```python
from build123d import *

# Parameters (mm, degrees)
SKETCH1_W           = 35
SKETCH1_H           = 10
BOSS_EXTRUDE1_DEPTH = 70
SKETCH2_3_R         = 7.5
SKETCH2_3_R_2       = 5
BOSS_EXTRUDE2_DEPTH = 10
CUT_EXTRUDE1_START  = -70
SKETCH2_4_R         = 5
CUT_EXTRUDE1_DEPTH  = 70
SKETCH3_R           = 7.5
SKETCH3_R_2         = 5
BOSS_EXTRUDE3_DEPTH = 10
CUT_EXTRUDE3_START  = -10
SKETCH3_2_R         = 5
CUT_EXTRUDE3_DEPTH  = 10
BOSS_EXTRUDE6_START = 6
BOSS_EXTRUDE6_DEPTH = 6


with BuildPart() as part:
    # Sketch1 → Revolve1 (revolve)
    with BuildSketch(Plane(origin=(0, 0, 0), x_dir=(0, 0, -1), z_dir=(1, 0, 0)), mode=Mode.PRIVATE) as revolve1_sk:
        Polygon((35, 79.538461538), (35, 89.538461538), (45, 89.538461538), (45, -20.461538462), (0, -20.461538462), (0, -10.461538462), (0, 49.538461538), (8, 49.538461538), (27, -10.461538462), (35, -10.461538462), align=None)
        with Locations((17.5, 84.538461538)):
            Rectangle(SKETCH1_W, SKETCH1_H)
    revolve(revolve1_sk.sketch.rotate(Axis((0, 0, 0), (0, -1, 0)), 180), axis=Axis((0, 0, 0), (0, -1, 0)))

    # Sketch2 → Boss-Extrude1 (add)
    with BuildSketch(Plane.XZ.offset(20.461538462)):
        with BuildLine():
            Line((40, 5), (10.356157589, 5))
            ThreePointArc((10.356157589, 5), (10.819851722, 3.896255731), (11.166285361, 2.750285665))
            Line((11.166285361, 2.750285665), (22.5, 1))
            Line((22.5, 1), (22.5, -1))
            Line((22.5, -1), (11.166285361, -2.750285665))
            ThreePointArc((11.166285361, -2.750285665), (10.819851722, -3.896255731), (10.356157589, -5))
            Line((10.356157589, -5), (40, -5))
            Line((40, -5), (40, 5))
        make_face()
        with BuildLine():
            ThreePointArc((2.750285665, 11.166285361), (3.896255731, 10.819851722), (5, 10.356157589))
            Line((5, 10.356157589), (5, 40))
            Line((5, 40), (-5, 40))
            Line((-5, 40), (-5, 10.356157589))
            ThreePointArc((-5, 10.356157589), (-3.896255731, 10.819851722), (-2.750285665, 11.166285361))
            Line((-2.750285665, 11.166285361), (-1, 22.5))
            Line((-1, 22.5), (1, 22.5))
            Line((1, 22.5), (2.750285665, 11.166285361))
        make_face()
        with BuildLine():
            Line((5, -40), (5, -10.356157589))
            ThreePointArc((5, -10.356157589), (3.896255731, -10.819851722), (2.750285665, -11.166285361))
            Line((2.750285665, -11.166285361), (1, -22.5))
            Line((1, -22.5), (-1, -22.5))
            Line((-1, -22.5), (-2.750285665, -11.166285361))
            ThreePointArc((-2.750285665, -11.166285361), (-3.896255731, -10.819851722), (-5, -10.356157589))
            Line((-5, -10.356157589), (-5, -40))
            Line((-5, -40), (5, -40))
        make_face()
        with BuildLine():
            ThreePointArc((-11.166285361, 2.750285665), (-10.819851722, 3.896255731), (-10.356157589, 5))
            Line((-10.356157589, 5), (-40, 5))
            Line((-40, 5), (-40, -5))
            Line((-40, -5), (-10.356157589, -5))
            ThreePointArc((-10.356157589, -5), (-10.819851722, -3.896255731), (-11.166285361, -2.750285665))
            Line((-11.166285361, -2.750285665), (-22.5, -1))
            Line((-22.5, -1), (-22.5, 1))
            Line((-22.5, 1), (-11.166285361, 2.750285665))
        make_face()
    extrude(amount=-BOSS_EXTRUDE1_DEPTH)

    # Sketch2<3> → Boss-Extrude2 (add)
    with BuildSketch(Plane.XZ.offset(20.461538462)):
        with Locations(Location((0, 0, 0), (0, 0, 270))):
            Circle(SKETCH2_3_R)
        with Locations(Location((0, 0, 0), (0, 0, 270))):
            Circle(SKETCH2_3_R_2, mode=Mode.SUBTRACT)
    extrude(amount=BOSS_EXTRUDE2_DEPTH)

    # Sketch2<4> → Cut-Extrude1 (cut)
    with BuildSketch(Plane.XZ.offset(20.461538462).offset(CUT_EXTRUDE1_START)):
        with Locations(Location((0, 0, 0), (0, 0, 270))):
            Circle(SKETCH2_4_R)
    extrude(amount=CUT_EXTRUDE1_DEPTH, mode=Mode.SUBTRACT)

    # Sketch3 → Boss-Extrude3 (add)
    with BuildSketch(Plane(origin=(0, 89.538461538, 0), x_dir=(1, 0, 0), z_dir=(0, 1, 0))):
        with Locations(Location((22, 0, 0), (0, 0, 270))):
            Circle(SKETCH3_R)
        with Locations(Location((22, 0, 0), (0, 0, 270))):
            Circle(SKETCH3_R_2, mode=Mode.SUBTRACT)
    extrude(amount=BOSS_EXTRUDE3_DEPTH)

    # Sketch3<2> → Cut-Extrude3 (cut)
    with BuildSketch(Plane(origin=(0, 89.538461538, 0), x_dir=(1, 0, 0), z_dir=(0, 1, 0)).offset(CUT_EXTRUDE3_START)):
        with Locations(Location((22, 0, 0), (0, 0, 270))):
            Circle(SKETCH3_2_R)
    extrude(amount=CUT_EXTRUDE3_DEPTH, mode=Mode.SUBTRACT)

    # Sketch2<5> → Boss-Extrude6 (add)
    with BuildSketch(Plane.XZ.offset(20.461538462).offset(BOSS_EXTRUDE6_START)):
        with BuildLine():
            ThreePointArc((-9.840501743, 5.951010455), (-8.131727984, 8.131727984), (-5.951010455, 9.840501743))
            Line((-5.951010455, 9.840501743), (-15.202795796, 16.617009358))
            Line((-15.202795796, 16.617009358), (-15.909902577, 15.909902577))
            Line((-15.909902577, 15.909902577), (-16.617009358, 15.202795796))
            Line((-16.617009358, 15.202795796), (-9.840501743, 5.951010455))
        make_face()
        with BuildLine():
            ThreePointArc((-2.750285665, 11.166285361), (0, 11.5), (2.750285665, 11.166285361))
            Line((2.750285665, 11.166285361), (1, 22.5))
            Line((1, 22.5), (0, 22.5))
            Line((0, 22.5), (-1, 22.5))
            Line((-1, 22.5), (-2.750285665, 11.166285361))
        make_face()
        with BuildLine():
            ThreePointArc((5.951010455, 9.840501743), (8.131727984, 8.131727984), (9.840501743, 5.951010455))
            Line((9.840501743, 5.951010455), (16.617009358, 15.202795796))
            Line((16.617009358, 15.202795796), (15.909902577, 15.909902577))
            Line((15.909902577, 15.909902577), (15.202795796, 16.617009358))
            Line((15.202795796, 16.617009358), (5.951010455, 9.840501743))
        make_face()
        with BuildLine():
            Line((22.5, 1), (11.166285361, 2.750285665))
            ThreePointArc((11.166285361, 2.750285665), (11.416266501, 1.385228925), (11.5, 0))
            ThreePointArc((11.5, 0), (11.416266501, -1.385228925), (11.166285361, -2.750285665))
            Line((11.166285361, -2.750285665), (22.5, -1))
            Line((22.5, -1), (22.5, 0))
            Line((22.5, 0), (22.5, 1))
        make_face()
        with BuildLine():
            Line((16.617009358, -15.202795796), (9.840501743, -5.951010455))
            ThreePointArc((9.840501743, -5.951010455), (8.131727984, -8.131727984), (5.951010455, -9.840501743))
            Line((5.951010455, -9.840501743), (15.202795796, -16.617009358))
            Line((15.202795796, -16.617009358), (15.909902577, -15.909902577))
            Line((15.909902577, -15.909902577), (16.617009358, -15.202795796))
        make_face()
        with BuildLine():
            Line((1, -22.5), (2.750285665, -11.166285361))
            ThreePointArc((2.750285665, -11.166285361), (0, -11.5), (-2.750285665, -11.166285361))
            Line((-2.750285665, -11.166285361), (-1, -22.5))
            Line((-1, -22.5), (0, -22.5))
            Line((0, -22.5), (1, -22.5))
        make_face()
        with BuildLine():
            Line((-15.202795796, -16.617009358), (-5.951010455, -9.840501743))
            ThreePointArc((-5.951010455, -9.840501743), (-8.131727984, -8.131727984), (-9.840501743, -5.951010455))
            Line((-9.840501743, -5.951010455), (-16.617009358, -15.202795796))
            Line((-16.617009358, -15.202795796), (-15.909902577, -15.909902577))
            Line((-15.909902577, -15.909902577), (-15.202795796, -16.617009358))
        make_face()
        with BuildLine():
            ThreePointArc((-11.166285361, -2.750285665), (-11.5, 0), (-11.166285361, 2.750285665))
            Line((-11.166285361, 2.750285665), (-22.5, 1))
            Line((-22.5, 1), (-22.5, 0))
            Line((-22.5, 0), (-22.5, -1))
            Line((-22.5, -1), (-11.166285361, -2.750285665))
        make_face()
    extrude(amount=-BOSS_EXTRUDE6_DEPTH)


solid = part.part
```
The model under review builds one solid part; all positions refer to its coordinate system, in mm. A direction names the side the tool comes from. Give positions to 0.01 mm unless a question says otherwise; leave off trailing zeros. Write each loop counter-clockwise with the first axis right and the second up, starting at its lowest first coordinate (ties: lowest second). Pieces come first, ordered by that corner, then holes. Notation, with made-up numbers: M 24.25,28.25 L 64.25,28.25 A22 cw 64.25,45.25 Z; hole C 34,-30.75 d8. An arc over 180 degrees is marked long. Write each question's results on one line, items separated by ' | '. Start each with the question number.
1. We need section A-A (y = 18). Count the separate pieces of the cut face and the enclosed holes in it, and give its area (3 significant figures).
2. We need section C-C (z = 37). Write out the cut boundary in (x, y).
3. For faces 5 (the flat face through (-16.912, -23.504, -1.863)), 6 (the flat face through (0, 49.538, -25)), 7 (the cylindrical face through (0, -23.5, -11.5)), list the 3-axis set-ups (+Z, -Z, +X, -X, +Y, -Y) from which the entire face can be reached by the end or side of a thin tool; tool diameter is ignored.
4. For probe 1 along Y at (x, z) = (-28, -11.5); probe 2 along X at (y, z) = (94.5, 0); probe 3 along X at (y, z) = (12, 0), list the stretches that pass through material, from the lowest coordinate up. Write a range as [from, to].
5. We need section D-D (z = -37.5). Write out the cut boundary in (x, y).
6. Insertion check: pin 1 Ø11 at (x, z) = (1.5, 21) entering from +Y; pin 2 Ø1.5 at (x, z) = (2, -17.5) entering from -Y; pin 3 Ø0.6 at (y, z) = (21.5, 0.5) entering from -X. Each pin has a flat end and moves straight along its axis. Give the tip position at first contact, or say it passes through.
7. We need section B-B (y = 56.5). Write out the cut boundary in (x, z), and give its area (3 significant figures).
8. Mouldability with a two-part tool opening along Z and no side actions: class faces 1 (the flat face through (-11, -26.462, 11)), 2 (the flat face through (-1.863, -23.504, 16.912)), 3 (the flat face through (-5, 26, -25)), 4 (the cylindrical face through (8.104, -23.504, 8.159)) as released by +Z, released by -Z, zero draft, split by the parting line, or undercut.
Results found:
1) separate pieces: 1 | enclosed holes: 9 | area: 4,090 mm^2
2) outline: M -25.61,-20.46 L 25.61,-20.46 L 25.61,89.54 L -25.61,89.54 Z
3) face 5: -X, -Y | face 6: none | face 7: -Y
4) probe 1: y = [-20.46, -10.46], [79.54, 89.54] | probe 2: x = [14.5, 17], [27, 29.5] | probe 3: x = [-45, -22.5], [-19.89, -5], [5, 19.89], [22.5, 45]
5) outline: M -24.87,-20.46 L 24.87,-20.46 L 24.87,89.54 L -24.87,89.54 Z
6) pin 1: stops at y = 89.54 | pin 2: stops at y = -26.46 | pin 3: stops at x = -45
7) outline: C 0,0 d90; hole C 0,0 d70 | area: 2,510 mm^2
8) face 1: zero draft | face 2: released by +Z | face 3: undercut | face 4: undercut
